```python
from build123d import *

# Parameters (mm, degrees)
F0_W     = 50
F0_H     = 100
F1_DEPTH = 25
F2_T     = -2
F3_W     = 12.5
F3_H     = 7
F3_W_2   = 8
F3_H_2   = 1.8
F4_DEPTH = 2
F5_R     = 3
F6_R     = 2.99999


# Not quite as in the source:
# - a fillet or chamfer is up to 0.001 mm smaller than in the source, because OpenCascade refuses the exact size


with BuildPart() as f1:
    # F0 (on Top) → F1 (new body)
    with BuildSketch(Plane.XY):
        Rectangle(F0_W, F0_H)
    extrude(amount=F1_DEPTH)

    # F2
    f2_openings = [f1.faces().sort_by_distance(p)[0] for p in [
        (0, 0, 25),
    ]]
    offset(amount=F2_T, openings=f2_openings)

    # F3 (on face) → F4 (cut)
    with BuildSketch(Plane.XZ.offset(50)):
        with Locations((14.25, 6.5)):
            Rectangle(F3_W, F3_H)
        with Locations((1, 3.9)):
            Rectangle(F3_W_2, F3_H_2)
    extrude(amount=-F4_DEPTH, mode=Mode.SUBTRACT)

    # F5
    f5_edges = [f1.edges().sort_by_distance(p)[0] for p in [
        (25, -50, 12.5),
    ]]
    fillet(f5_edges, radius=F5_R)

    # F6 (radius 3 in the source; OpenCascade refuses exactly that, so slightly less here)
    f6_edges = [f1.edges().sort_by_distance(p)[0] for p in [
        (25, 50, 12.5),
        (-25, 50, 12.5),
        (-25, -50, 12.5),
        (-25, 0, 0),
        (-1.5, -50, 0),
        (0, 50, 0),
    ]]
    fillet(f6_edges, radius=F6_R)


solid = f1.part
```
Input: part model. Units: mm. Frame: model coordinates. A direction names the side the tool comes from. Coordinates: 2 decimals unless noted, no trailing zeros. Loops run counter-clockwise (first coordinate to the right, second up) from the corner with the lowest first, then second, coordinate; pieces in that order, holes last. Notation, with made-up numbers: M 42,46.25 L 53,46.25 A27 ccw 53,74.25 Z; hole C -16.5,73.5 d11. An arc over 180 degrees is marked long. Use a Markdown table: item, result. Add a question column.
1) Pin query (flat end, axial travel): P1, Ø1.4, axis at y = -49.5, z = 4, coming from the +X side; P2, Ø1.6, axis at x = 12.5, y = -48.5, coming from the -Z side; P3, Ø1.5, axis at x = -11, y = 6.5, coming from the +Z side; P4, Ø6, axis at x = -0.5, y = 2.5, coming from the -Z side. Return the tip coordinate at first contact, or that it passes through.
2) Section D-D, the plane z = 5.75. Return the cut outline in (x, y), plus the area to 3 significant figures.
3) Line query: L1, parallel to Y at x = 8, z = 23.5; L2, parallel to X at y = 1.5, z = 4.75; L3, parallel to Z at x = 7, y = -5. Output: solid intervals per line, ascending. Write a range as from..to.
4) Section C-C, the plane y = -13. Return the cut outline in (x, z).
5) Set-up query: faces 1 (the cylindrical face through (-24.1, -49.14, 14.15)), 2 (the flat face through (0, 48, 13)), 3 (the flat face through (20.5, -49, 6)). Return all of +Z, -Z, +X, -X, +Y, -Y with unobstructed straight access to the full face (end or side cutting, diameter ignored); none if empty.
6) Draft query along Y for faces 4 (the flat face through (0, -48, 16)), 5 (the cylindrical face through (0.31, 49.1, 0.86)), 6 (the flat face through (-3, -49, 4)), 7 (the flat face through (0, -50, 14)). Return one class per face: +Y half, -Y half, draft (parallel to the pull), parting line (faces both ways), or undercut.
7) Section A-A, the plane z = 16.25. Return the cut outline in (x, y).
Answer below:
| question | item | result |
|---|---|---|
| 1 | P1 | x = 24.4 |
| 1 | P2 | z = 0.08 |
| 1 | P3 | z = 2 |
| 1 | P4 | z = 0 |
| 2 | outline | M -25,-47 A3 ccw -22,-50 L 8,-50 L 8,-48 L -23,-48 L -23,48 L 23,48 L 23,-48 L 20.5,-48 L 20.5,-50 L 22,-50 A3 ccw 25,-47 L 25,47 A3 ccw 22,50 L -22,50 A3 ccw -25,47 Z |
| 2 | area | 551 mm2 |
| 3 | L1 | -50..-48, 48..50 |
| 3 | L2 | -25..-23, 23..25 |
| 3 | L3 | 0..2 |
| 4 | outline | M -25,3 A3 ccw -22,0 L 22,0 A3 ccw 25,3 L 25,25 L 23,25 L 23,2 L -23,2 L -23,25 L -25,25 Z |
| 5 | face 1 | +Z, -Z, -X, -Y |
| 5 | face 2 | +Z |
| 5 | face 3 | -Y |
| 6 | face 4 | undercut |
| 6 | face 5 | +Y half |
| 6 | face 6 | draft |
| 6 | face 7 | -Y half |
| 7 | outline | M -25,-47 A3 ccw -22,-50 L 22,-50 A3 ccw 25,-47 L 25,47 A3 ccw 22,50 L -22,50 A3 ccw -25,47 Z; hole M -23,-48 L 23,-48 L 23,48 L -23,48 Z |
